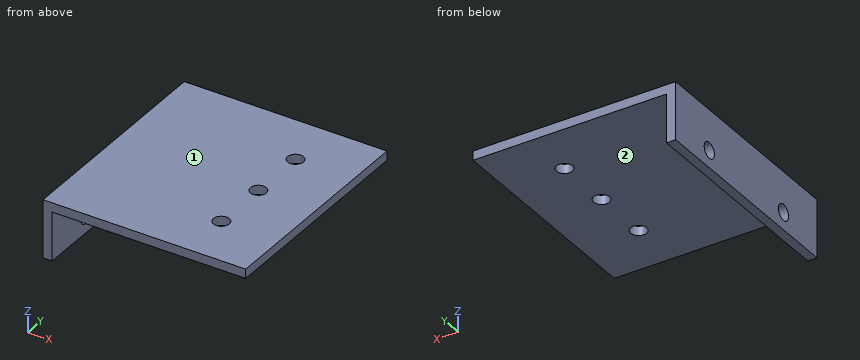
```python
from build123d import *

# Parameters (mm, degrees)
EXTRUDE_THIN1_DEPTH  = 38.1
M5_CLEARANCE_HOLE1_D = 5.5
M5_CLEARANCE_HOLE2_D = 5.5


with BuildPart() as part:
    # Sketch1 → Extrude-Thin1 (new body, symmetric)
    with BuildSketch(Plane(origin=(0, 0, 0), x_dir=(1, 0, 0), z_dir=(0, 1, 0))):
        Polygon((0, 20), (0, 0), (70, 0), (70, 3.175), (3.175, 3.175), (3.175, 20), align=None)
    extrude(amount=EXTRUDE_THIN1_DEPTH, both=True)

    # M5 Clearance Hole1 (through all)
    with Locations(Plane.XY):
        with Locations((50, 20), (50, 0), (50, -20)):
            Hole(M5_CLEARANCE_HOLE1_D / 2)

    # M5 Clearance Hole2 (through all)
    with Locations(Plane(origin=(3.175, 0, 0), x_dir=(0, 0, -1), z_dir=(1, 0, 0))):
        with Locations((14, 20), (14, -20)):
            Hole(M5_CLEARANCE_HOLE2_D / 2)


solid = part.part
```
Could you check a few things on this model? Use its own coordinates, in mm. Face numbers are marked on the shaded views. A direction names the side the tool comes from. Round coordinates to 2 decimals unless told otherwise and drop trailing zeros. Loops run counter-clockwise (first coordinate to the right, second up) from the corner with the lowest first, then second, coordinate; pieces in that order, holes last. Notation, with made-up numbers: (0, -9) -> (52, -9) arc R16 ccw to (52, -2) -> close; hole circle Ø4 at (80, 61.5). An arc over 180 degrees is marked (long way). Put each result on its own line as item: value.
Q1. I want a section at D-D on y = 20. Write out the boundary of the cut face in (x, z) (3 decimals).
Checks:
outline: (0, -20) -> (3.175, -20) -> (3.175, -16.75) -> (0, -16.75) -> close; (0, -11.25) -> (3.175, -11.25) -> (3.175, -3.175) -> (47.25, -3.175) -> (47.25, 0) -> (0, 0) -> close; (52.75, -3.175) -> (70, -3.175) -> (70, 0) -> (52.75, 0) -> close
Q2. Which directions (+Z, -Z, +X, -X, +Y, -Y) give clear straight access to the entire face, cutting with the end or side of a thin tool? Please do the marked faces 1 and 2.
Checks:
face 1: +Z, +X, -X, +Y, -Y
face 2: -Z, +X, +Y, -Y
Q3. I want a section at B-B on y = 0. Write out the boundary of the cut face in (x, z) (3 decimals), and give its area (3 significant figures).
Checks:
outline: (0, -20) -> (3.175, -20) -> (3.175, -3.175) -> (47.25, -3.175) -> (47.25, 0) -> (0, 0) -> close; (52.75, -3.175) -> (70, -3.175) -> (70, 0) -> (52.75, 0) -> close
area: 258 mm2
Q4. I want a section at A-A on x = 50. Write out the boundary of the cut face in (y, z) (3 decimals).
Checks:
outline: (-38.1, -3.175) -> (-22.75, -3.175) -> (-22.75, 0) -> (-38.1, 0) -> close; (-17.25, -3.175) -> (-2.75, -3.175) -> (-2.75, 0) -> (-17.25, 0) -> close; (2.75, -3.175) -> (17.25, -3.175) -> (17.25, 0) -> (2.75, 0) -> close; (22.75, -3.175) -> (38.1, -3.175) -> (38.1, 0) -> (22.75, 0) -> close
Q5. For pin 1 Ø2 at (x, y) = (54.5, 19.5) entering from -Z (3 decimals); pin 2 Ø5 at (y, z) = (15, -11.5) entering from +X (3 decimals), each with a flat end and sliding along its axis, tell me the tip position at first contact or that it passes through.
Checks:
pin 1: z = -3.175
pin 2: x = 3.175
Q6. I want a section at C-C on z = -14. Write out the boundary of the cut face in (x, y) (3 decimals), and give its area (3 significant figures).
Checks:
outline: (0, -38.1) -> (3.175, -38.1) -> (3.175, -22.75) -> (0, -22.75) -> close; (0, -17.25) -> (3.175, -17.25) -> (3.175, 17.25) -> (0, 17.25) -> close; (0, 22.75) -> (3.175, 22.75) -> (3.175, 38.1) -> (0, 38.1) -> close
area: 207 mm2
Q7. Please list where these lines run through material, in increasing order: line 1 (Y direction, x = 50, z = -1.05); line 2 (Y direction, x = 2.5, z = -14); line 3 (Z direction, x = 57, y = -7) (3 decimals). Write a range as from..to.
Checks:
line 1: -38.1..-22.75, -17.25..-2.75, 2.75..17.25, 22.75..38.1
line 2: -38.1..-22.75, -17.25..17.25, 22.75..38.1
line 3: -3.175..0
